The figure shows three views and two pictorial views of one solid part (mm, origin at its lowest corner). Answer the questions. A direction names the side the tool comes from. Round coordinates to 2 decimals unless told otherwise and drop trailing zeros. Write each loop counter-clockwise with the first axis right and the second up, starting at its lowest first coordinate (ties: lowest second). Pieces come first, ordered by that corner, then holes. Notation, with made-up numbers: M 11.5,21 L 58.5,21 A16 cw 58.5,26 Z; hole C -25.75,84.25 d10. An arc over 180 degrees is marked long. One line per item, written item: value. Start each with the question number.
Q1. Find section B-B (y = 13). Write down the section's boundary in (x, z).
Q2. Given pin 1 Ø3 at (y, z) = (2.5, 4) entering from -X; pin 2 Ø1.1 at (y, z) = (40, 2) entering from -X; pin 3 Ø3 at (y, z) = (20, 3) entering from +X; pin 4 Ø3 at (x, z) = (36, 4.5) entering from -Y (3 decimals), each flat-ended and moving along its own axis, determine where each tip first touches the part or whether it passes through.
Q3. Find section C-C (z = 5.45). Write down the section's boundary in (x, y) (3 decimals), and give its area (3 significant figures).
Q4. Find section A-A (x = 34.5). Write down the section's boundary in (y, z) (3 decimals), and give its area (3 significant figures).
Q5. A tool of negligible diameter and unlimited length cuts with its end or side. For the marked faces 1, 2 and 3, from which of +Z, -Z, +X, -X, +Y, -Y can it reach the whole face along a straight path? Write none if from no direction.
Q6. Consider probe 1 along X at (y, z) = (10.5, 4.65); probe 2 along X at (y, z) = (9, 3.2); probe 3 along Y at (x, z) = (20, 4). Determine where each line is inside the solid, lowest interval first.
Q7. The mould has two halves that part along Y. Classify the marked faces 4, 5 and 6: released by +Y, released by -Y, zero draft, split by the parting line, or undercut.
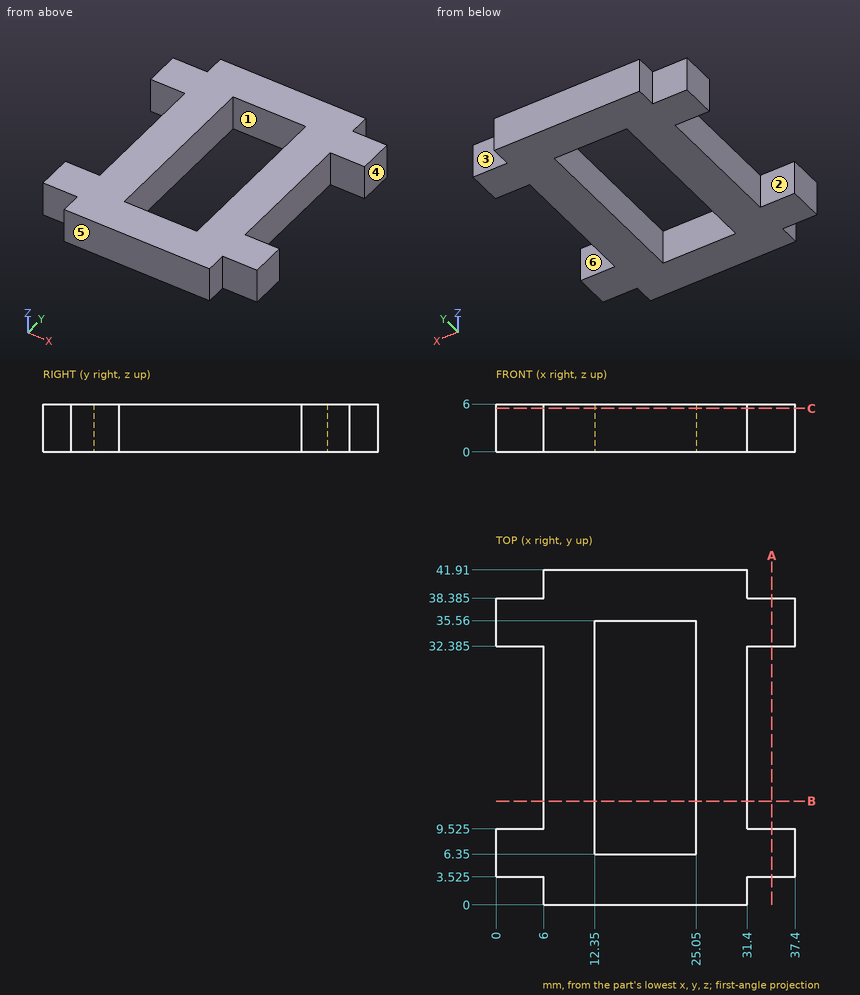
The answers:
1. outline: M 6,0 L 12.35,0 L 12.35,6 L 6,6 Z; M 25.05,0 L 31.4,0 L 31.4,6 L 25.05,6 Z
2. pin 1: x = 0
2. pin 2: x = 6
2. pin 3: x = 31.4
2. pin 4: y = 3.525
3. outline: M 0,3.525 L 6,3.525 L 6,0 L 31.4,0 L 31.4,3.525 L 37.4,3.525 L 37.4,9.525 L 31.4,9.525 L 31.4,32.385 L 37.4,32.385 L 37.4,38.385 L 31.4,38.385 L 31.4,41.91 L 6,41.91 L 6,38.385 L 0,38.385 L 0,32.385 L 6,32.385 L 6,9.525 L 0,9.525 Z; hole M 12.35,6.35 L 25.05,6.35 L 25.05,35.56 L 12.35,35.56 Z
3. area: 838 mm2
4. outline: M 3.525,0 L 9.525,0 L 9.525,6 L 3.525,6 Z; M 32.385,0 L 38.385,0 L 38.385,6 L 32.385,6 Z
4. area: 72.0 mm2
5. face 1: +Z, -Z
5. face 2: +Z, -Z, -X
5. face 3: +Z, -Z, +X, +Y
6. probe 1: 6 to 12.35, 25.05 to 31.4
6. probe 2: 0 to 12.35, 25.05 to 37.4
6. probe 3: 0 to 6.35, 35.56 to 41.91
7. face 4: zero draft
7. face 5: released by -Y
7. face 6: undercut
